```python
from build123d import *

# Parameters (mm, degrees)
SKETCH1_W           = 28.24
SKETCH1_H           = 80
BOSS_EXTRUDE1_DEPTH = 3
SKETCH3_W           = 28.24
SKETCH3_H           = 10
BOSS_EXTRUDE3_DEPTH = 3
CUT_EXTRUDE1_REACH  = 54.042
SKETCH4_R           = 2.5


with BuildPart() as part:
    # Sketch1 → Boss-Extrude1 (new body)
    with BuildSketch(Plane.XY):
        Rectangle(SKETCH1_W, SKETCH1_H)
    extrude(amount=BOSS_EXTRUDE1_DEPTH)

    # Sketch3 → Boss-Extrude3 (add)
    with BuildSketch(Plane(origin=(0, 0, 0), x_dir=(-1, 0, 0), z_dir=(0, 0, -1))):
        with Locations((0, 45)):
            Rectangle(SKETCH3_W, SKETCH3_H)
    extrude(amount=-BOSS_EXTRUDE3_DEPTH)

    # Sketch4 → Cut-Extrude1 (cut, up to next)
    with BuildSketch(Plane(origin=(0, 0, 0), x_dir=(-1, 0, 0), z_dir=(0, 0, -1)), mode=Mode.PRIVATE) as cut_extrude1_sk1:
        with Locations((9.12, 45)):
            Circle(SKETCH4_R)
    cut_extrude1_tool1 = extrude(cut_extrude1_sk1.sketch, amount=-CUT_EXTRUDE1_REACH, mode=Mode.PRIVATE) & part.part
    cut_extrude1 = cut_extrude1_tool1.solids().sort_by_distance((-9.12, 45, 0))[0]
    add(cut_extrude1, mode=Mode.SUBTRACT)

    # Mirror1: Cut-Extrude1 across plane
    add(cut_extrude1.mirror(Plane(origin=(0, 0, 0), x_dir=(0, 0, 1), z_dir=(1, 0, 0))), mode=Mode.SUBTRACT)


solid = part.part
```
Build history of the part. All positions in model axes, mm. Round coordinates to 2 decimals unless told otherwise and drop trailing zeros. Write each loop counter-clockwise with the first axis right and the second up, starting at its lowest first coordinate (ties: lowest second). Pieces come first, ordered by that corner, then holes.
1) Mould opens along X. For faces 1 (the flat face through (0, -40, 1)), 2 (the cylindrical face through (8.58, 42.56, 1.48)), 3 (the flat face through (-14.12, 4, 1)), 4 (the flat face through (14.12, 4, 1)) say: +X half, -X half, draft (parallel to the pull), parting line (faces both ways), or undercut.
2) Band-saw the part on C-C, the plane z = 0.7. List the corners of the cut face in (x, y), and give its area (3 significant figures).
3) Band-saw the part on B-B, the plane y = 45. List the corners of the cut face in (x, z).
4) Band-saw the part on A-A, the plane x = 9.12. List the corners of the cut face in (y, z).
5) Pin check, flat tips, straight feed: pin 1 (10 mm diameter, centred on x = 5.5, y = -30.5, fed in from -Z); pin 2 (4 mm diameter, centred on x = -9.12, y = 45, fed in from -Z). Stop position of each tip, or through.
6) Drill centre lines: probe 1 along Y at (x, z) = (9.12, 2.05); probe 2 along Y at (x, z) = (11.25, 2.25). Where is each one in solid material? Low to high.
Ans:
1. face 1: draft
1. face 2: undercut
1. face 3: -X half
1. face 4: +X half
2. outline: (-14.12, -40) - (14.12, -40) - (14.12, 50) - (-14.12, 50) - close; hole circle Ø5 at (-9.12, 45); hole circle Ø5 at (9.12, 45)
2. area: 2,500 mm2
3. outline: (-14.12, 0) - (-11.62, 0) - (-11.62, 3) - (-14.12, 3) - close; (-6.62, 0) - (6.62, 0) - (6.62, 3) - (-6.62, 3) - close; (11.62, 0) - (14.12, 0) - (14.12, 3) - (11.62, 3) - close
4. outline: (-40, 0) - (42.5, 0) - (42.5, 3) - (-40, 3) - close; (47.5, 0) - (50, 0) - (50, 3) - (47.5, 3) - close
5. pin 1: stops at z = 0
5. pin 2: passes through
6. probe 1: y = -40 to 42.5, 47.5 to 50
6. probe 2: y = -40 to 43.69, 46.31 to 50
